The model under review builds one solid part; all positions refer to its coordinate system, in mm. Face numbers are marked on the shaded views. A direction names the side the tool comes from. Coordinates: 2 decimals unless noted, no trailing zeros. Order: outer loops, then holes, each group sorted by start corner. A loop starts at its lowest first (then second) coordinate and runs counter-clockwise, first axis right, second up. Notation, with made-up numbers: (-5.5, 49) -> (23.5, 49) arc R28 ccw to (23.5, 83) -> close; hole circle Ø7 at (62, 81.5). An arc over 180 degrees is marked (long way). Use one line per item in the form item = value. Start each with the question number.
(1) Take a section at C-C (x = 0). State the section outline as (y, z) points, then the cut area to 3 significant figures.
(2) Take a section at B-B (z = 52.5). State the section outline as (x, y) points.
(3) For the marked faces 1 and 2, list the 3-axis set-ups (+Z, -Z, +X, -X, +Y, -Y) from which the entire face can be reached by the end or side of a thin tool; tool diameter is ignored.
(4) Wall thickness on line 1 along Z through (x, y) = (0, 12.35); line 2 along X through (y, z) = (-1, 157); line 3 along Y through (x, z) = (-3, 70): over which ranges is each line inside the solid? List them lowest first.
(5) Take a section at A-A (y = 6.5). State the section outline as (x, z) points, then the cut area to 3 significant figures.
(6) Take a section at D-D (z = 106.68). State the section outline as (x, y) points, then the cut area to 3 significant figures.
(7) Insertion check: pin 1 Ø4.5 at (x, z) = (17.526, 89.154) entering from +Y. The pin has a flat end and moves straight along its axis. Give the tip position at first contact, or say it passes through.
(8) Mouldability with a two-part tool opening along X and no side actions: class the marked faces 3, 4, 5 and 6 as +X half, -X half, draft (parallel to the pull), parting line (faces both ways), or undercut.
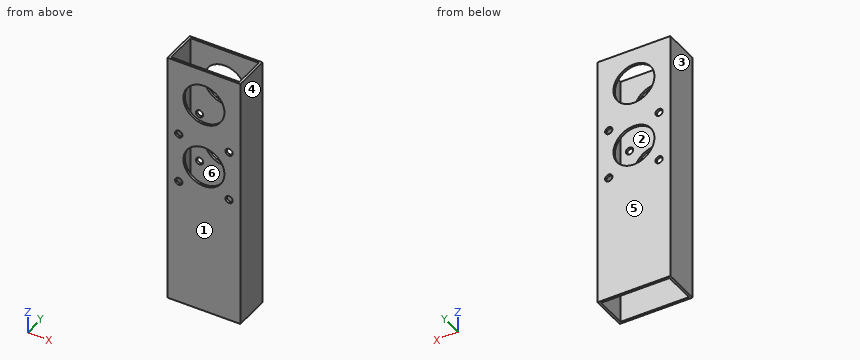
```python
from build123d import *

# Parameters (mm, degrees)
F0_W     = 50.8
F0_H     = 25.4
F0_W_2   = 47.625
F0_H_2   = 22.225
F1_DEPTH = 177.8
F2_R     = 14.2875
F2_R_2   = 2.5527
F3_DEPTH = 25.4


with BuildPart() as f1:
    # F0 (on Top) → F1 (new body)
    with BuildSketch(Plane.XY):
        Rectangle(F0_W, F0_H)
        Rectangle(F0_W_2, F0_H_2, mode=Mode.SUBTRACT)
    extrude(amount=F1_DEPTH)

    # F2 (on face) → F3 (cut)
    with BuildSketch(Plane.XZ.offset(12.7)):
        with Locations((0, 152.4)):
            Circle(F2_R)
        with Locations((-17.526, 124.206)):
            Circle(F2_R_2)
        with Locations((17.526, 124.206)):
            Circle(F2_R_2)
        with Locations((17.526, 89.154)):
            Circle(F2_R_2)
        with Locations((-17.526, 89.154)):
            Circle(F2_R_2)
        with Locations((0, 106.68)):
            Circle(F2_R)
    extrude(amount=-F3_DEPTH, mode=Mode.SUBTRACT)


solid = f1.part
```
Findings:
q1.outline = (-12.7, 0) -> (-11.11, 0) -> (-11.11, 92.39) -> (-12.7, 92.39) -> close; (-12.7, 120.97) -> (-11.11, 120.97) -> (-11.11, 138.11) -> (-12.7, 138.11) -> close; (-12.7, 166.69) -> (-11.11, 166.69) -> (-11.11, 177.8) -> (-12.7, 177.8) -> close; (11.11, 0) -> (12.7, 0) -> (12.7, 92.39) -> (11.11, 92.39) -> close; (11.11, 120.97) -> (12.7, 120.97) -> (12.7, 138.11) -> (11.11, 138.11) -> close; (11.11, 166.69) -> (12.7, 166.69) -> (12.7, 177.8) -> (11.11, 177.8) -> close
q1.area = 383 mm²
q2.outline = (-25.4, -12.7) -> (25.4, -12.7) -> (25.4, 12.7) -> (-25.4, 12.7) -> close; hole (-23.81, -11.11) -> (23.81, -11.11) -> (23.81, 11.11) -> (-23.81, 11.11) -> close
q3.face_1 = +Z, -Z, +X, -X, -Y
q3.face_2 = +Z, -Z
q4.line_1 = 0 to 92.39, 120.97 to 138.11, 166.69 to 177.8
q4.line_2 = -25.4 to -23.81, 23.81 to 25.4
q4.line_3 = -12.7 to -11.11, 11.11 to 12.7
q5.outline = (-25.4, 0) -> (-23.81, 0) -> (-23.81, 177.8) -> (-25.4, 177.8) -> close; (23.81, 0) -> (25.4, 0) -> (25.4, 177.8) -> (23.81, 177.8) -> close
q5.area = 565 mm²
q6.outline = (-25.4, -12.7) -> (-14.29, -12.7) -> (-14.29, -11.11) -> (-23.81, -11.11) -> (-23.81, 11.11) -> (-14.29, 11.11) -> (-14.29, 12.7) -> (-25.4, 12.7) -> close; (14.29, -12.7) -> (25.4, -12.7) -> (25.4, 12.7) -> (14.29, 12.7) -> (14.29, 11.11) -> (23.81, 11.11) -> (23.81, -11.11) -> (14.29, -11.11) -> close
q6.area = 141 mm²
q7.pin_1 = through
q8.face_3 = -X half
q8.face_4 = +X half
q8.face_5 = draft
q8.face_6 = undercut
